For this review, use the dimensioned drawing (mm, ordinates from the lowest corner) and the shaded views. A direction names the side the tool comes from. Coordinates: 2 decimals unless noted, no trailing zeros. Order: outer loops, then holes, each group sorted by start corner. A loop starts at its lowest first (then second) coordinate and runs counter-clockwise, first axis right, second up. Notation, with made-up numbers: M -6,83.25 L -1,83.25 A20 ccw -1,90.25 Z; hole C 31.5,62.5 d10. An arc over 180 degrees is marked long. Answer as CSV lines item,"result". Start each with the question number.
Q1. For P1, Ø2.5, axis at y = 10.5, z = 4.5, coming from the +X side; P2, Ø1.5, axis at x = 5, z = 4, coming from the +Y side, all flat-tipped, find the tip position at first contact; note any pin that passes through.
Q2. Consider section A-A on x = 9. Write out the cut boundary in (y, z).
Q3. Consider section C-C on y = 1.25. Write out the cut boundary in (x, z).
Q4. The part is to be moulded in two halves that separate along Y. For the marked faces 1, 2 and 3, say which applies: +Y half, -Y half, draft (parallel to the pull), parting line (faces both ways), or undercut.
Q5. Wall thickness on L1, parallel to X at y = 1.05, z = 4; L2, parallel to X at y = 14, z = 0.5: over which ranges is each line inside the solid? List them lowest first. Write a range as [from, to].
Q6. Consider section D-D on z = 7. Write out the cut boundary in (x, y).
Q7. Machinability: for the marked faces 4 and 5, which of the approach directions +Z, -Z, +X, -X, +Y, -Y give a long, thin tool a straight path to every point of the face, cutting with its end or side? Answer none if there is none.
Q8. Consider section B-B on z = 4. Write out the cut boundary in (x, y).
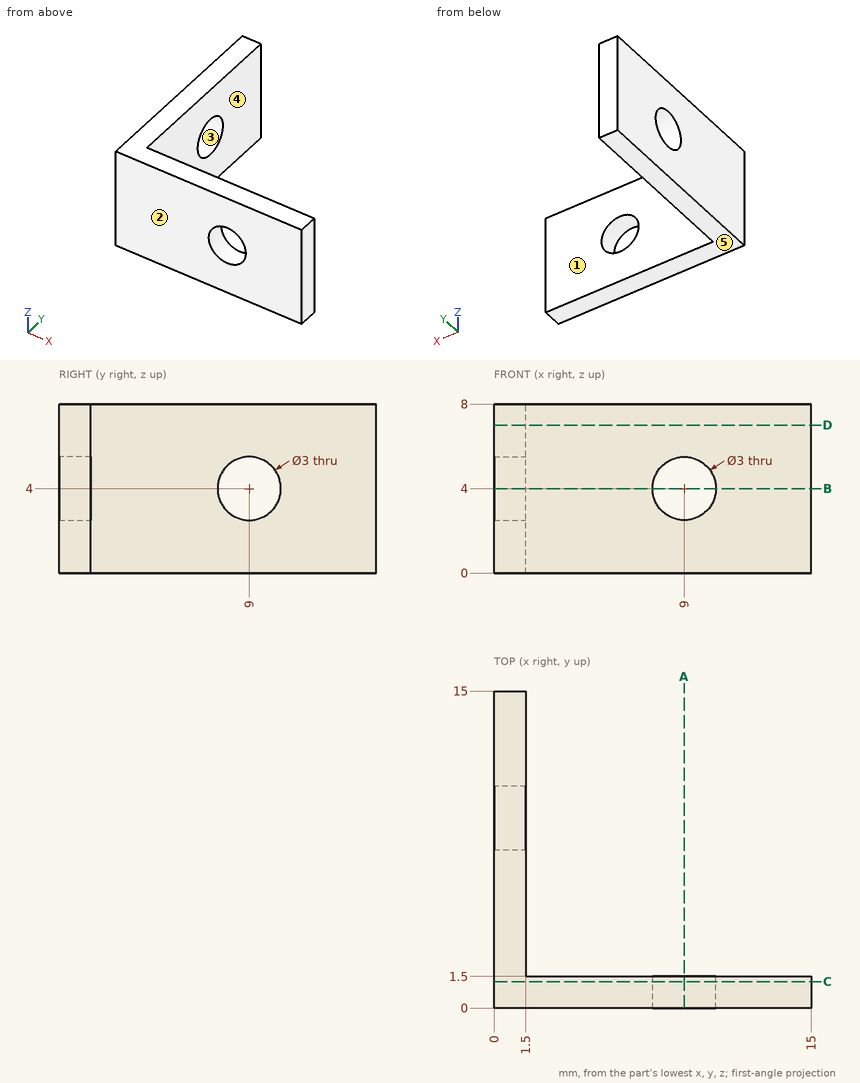
Evaluation:
1,P1,"stops at x = 1.5"
1,P2,"stops at y = 1.5"
2,outline,"M 0,0 L 1.5,0 L 1.5,2.5 L 0,2.5 Z; M 0,5.5 L 1.5,5.5 L 1.5,8 L 0,8 Z"
3,outline,"M 0,0 L 15,0 L 15,8 L 0,8 Z; hole C 9,4 d3"
4,face 1,"+Y half"
4,face 2,"-Y half"
4,face 3,"undercut"
5,L1,"x = [0, 7.5], [10.5, 15]"
5,L2,"x = [0, 1.5]"
6,outline,"M 0,0 L 15,0 L 15,1.5 L 1.5,1.5 L 1.5,15 L 0,15 Z"
7,face 4,"+Z, -Z, +X, +Y"
7,face 5,"-Z, +X, -X, +Y, -Y"
8,outline,"M 0,0 L 7.5,0 L 7.5,1.5 L 1.5,1.5 L 1.5,7.5 L 0,7.5 Z; M 0,10.5 L 1.5,10.5 L 1.5,15 L 0,15 Z; M 10.5,0 L 15,0 L 15,1.5 L 10.5,1.5 Z"
